```python
from build123d import *

# Parameters (mm, degrees)
F1_DEPTH = 2
F2_SIZE2 = 0.79999
F2_SIZE  = 1.99999


# Not quite as in the source:
# - a fillet or chamfer is up to 0.001 mm smaller than in the source, because OpenCascade refuses the exact size


with BuildPart() as f1:
    # F0 (on Top) → F1 (new body)
    with BuildSketch(Plane.XY):
        Polygon((-7.25, 4.1857894516), (-7.25, -4.1857894516), (0, -8.3715789032), (7.25, -4.1857894516), (7.25, 4.1857894516), (0, 8.3715789032), align=None)
        Polygon((0, 3.7527767497), (3.25, 1.8763883749), (3.25, -1.8763883749), (0, -3.7527767497), (-3.25, -1.8763883749), (-3.25, 1.8763883749), align=None, mode=Mode.SUBTRACT)
    extrude(amount=F1_DEPTH)

    # F2 (size 2 and 0.8 in the source; OpenCascade refuses exactly that, so slightly less here)
    f2_edges = [f1.edges().sort_by_distance(p)[0] for p in [
        (-7.25, 0, 2),
        (-3.625, -6.278684, 2),
        (3.625, -6.278684, 2),
        (7.25, 0, 2),
        (3.625, 6.278684, 2),
        (-3.625, 6.278684, 2),
        (-3.25, 0, 2),
        (-1.625, 2.814583, 2),
        (1.625, 2.814583, 2),
        (3.25, 0, 2),
        (1.625, -2.814583, 2),
        (-1.625, -2.814583, 2),
    ]]
    chamfer(f2_edges, length=F2_SIZE, length2=F2_SIZE2)


solid = f1.part
```
Part model, mm, in its own coordinate system. A direction names the side the tool comes from. Coordinates: 2 decimals unless noted, no trailing zeros. Order: outer loops, then holes, each group sorted by start corner. A loop starts at its lowest first (then second) coordinate and runs counter-clockwise, first axis right, second up. Notation, with made-up numbers: (38.5, -1.75) - (86.5, -1.75) arc R15 ccw to (86.5, 3.25) - close; hole circle Ø10 at (44, 23). An arc over 180 degrees is marked (long way). Return JSON: item names as keys, results as strings. Group by question number.
Item 1: Which spindle directions (+Z, -Z, +X, -X, +Y, -Y) get a long thin tool onto all of the face, cutting with end or side? Do faces 4 (the face through (1.8, 3.18, 1.01)), 5 (the face through (6.844, -0.059, 1.014)). Say none if no direction does.
Item 2: Drill centre lines: probe 1 along Y at (x, z) = (-0.5, 1); probe 2 along Y at (x, z) = (-0.5, 0.9); probe 3 along X at (y, z) = (-2.5, 0.35). Where is each one in solid material? Low to high. Write a range as from..to.
Item 3: Cut at D-D (z = 1.75). List the corners of the cut face in (x, y), plus the area to 3 significant figures.
Item 4: Cut at C-C (z = 0.45). List the corners of the cut face in (x, y).
Item 5: Pull direction Y, two halves, no side cores. Call faces 1 (the face through (3.656, 0.033, 1.014)), 2 (the face through (3.47, 5.9, 1.01)), 3 (the face through (-3, -3.2, 2)): pulls with the +Y half, pulls with the -Y half, needs draft (parallel to the pull), parting line crosses it, or undercut.
Check values:
{
 "1": {"face 4": "+Z", "face 5": "+Z, +X, +Y, -Y"},
 "2": {"probe 1": "y = -7.62..-3.93, 3.93..7.62", "probe 2": "y = -7.67..-3.88, 3.88..7.67", "probe 3": "x = -7.11..-2.45, 2.45..7.11"},
 "3": {"outline": "(-6.55, -3.78) - (0, -7.56) - (6.55, -3.78) - (6.55, 3.78) - (0, 7.56) - (-6.55, 3.78) - close; hole (-3.95, -2.28) - (0, -4.56) - (3.95, -2.28) - (3.95, 2.28) - (0, 4.56) - (-3.95, 2.28) - close", "area": "94.6 mm2"},
 "4": {"outline": "(-7.07, -4.08) - (0, -8.16) - (7.07, -4.08) - (7.07, 4.08) - (0, 8.16) - (-7.07, 4.08) - close; hole (-3.43, -1.98) - (0, -3.96) - (3.43, -1.98) - (3.43, 1.98) - (0, 3.96) - (-3.43, 1.98) - close"},
 "5": {"face 1": "undercut", "face 2": "pulls with the +Y half", "face 3": "needs draft"}
}
